Answer from the drawing. Dimensions are ordinates in mm from the lowest x, y and z of the part. Give positions to 0.01 mm unless a question says otherwise; leave off trailing zeros. Write each loop counter-clockwise with the first axis right and the second up, starting at its lowest first coordinate (ties: lowest second). Pieces come first, ordered by that corner, then holes.
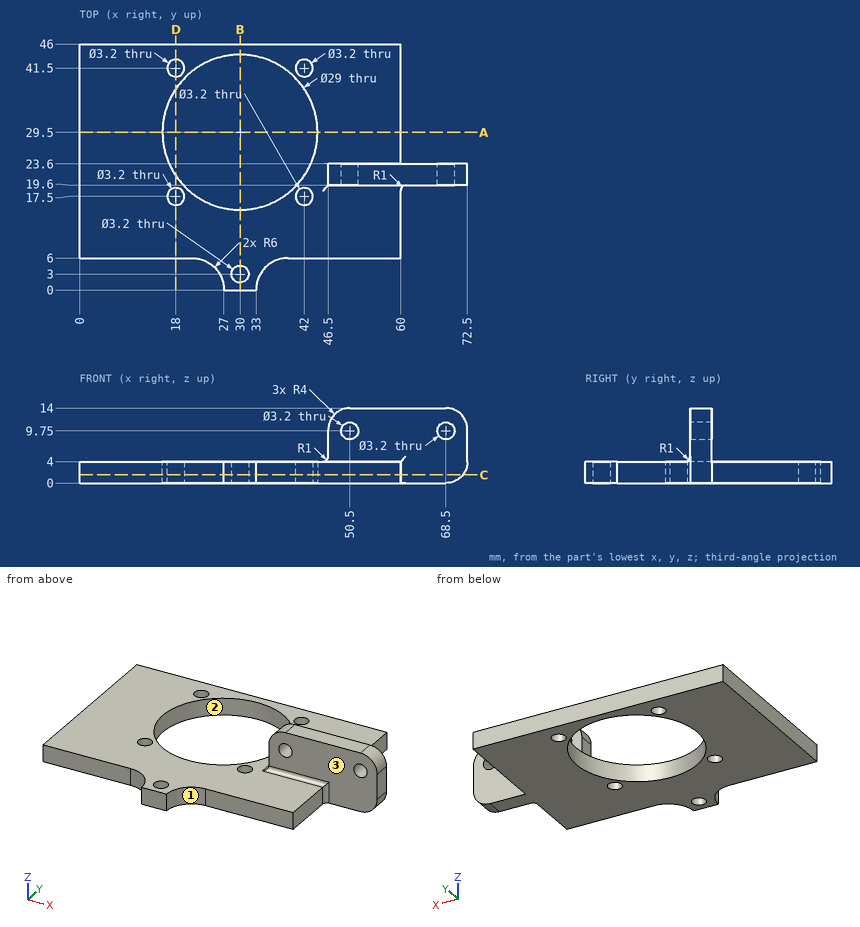
Item 1: A cutting plane is placed at C-C, the plane z = 1.5. Count the separate pieces of the cut face and the enclosed holes in it, plus the area to 3 significant figures.
Conclusion:
separate pieces: 1
enclosed holes: 6
area: 1,800 mm2
Item 2: Each of these flat-tipped pins is pushed along its axis until it touches: P1, Ø5, axis at x = 42, y = 41.5, coming from the +Z side; P2, Ø1.5, axis at y = 24, z = 3, coming from the +X side; P3, Ø2, axis at y = 34, z = 1, coming from the +X side. Where does it stop, or does it pass through?
Conclusion:
P1: stops at z = 4
P2: stops at x = 72.48
P3: stops at x = 60
Item 3: Consider probe 1 along Y at (x, z) = (30, 2.25); probe 2 along X at (y, z) = (22.15, 9.75); probe 3 along Y at (x, z) = (42, 1.9). Determine where each line is inside the solid, lowest interval first.
Conclusion:
probe 1: y = 0 to 1.4, 4.6 to 15, 44 to 46
probe 2: x = 46.5 to 48.9, 52.1 to 66.9, 70.1 to 72.5
probe 3: y = 6 to 15.9, 19.1 to 21.36, 37.64 to 39.9, 43.1 to 46
Item 4: A cutting plane is placed at A-A, the plane y = 29.5. Give the vertices of the cut face in (x, z), plus the area to 3 significant figures.
Conclusion:
outline: (0, 0) - (15.5, 0) - (15.5, 4) - (0, 4) - close; (44.5, 0) - (60, 0) - (60, 4) - (44.5, 4) - close
area: 124 mm2
Item 5: A cutting plane is placed at B-B, the plane x = 30. Give the vertices of the cut face in (y, z).
Conclusion:
outline: (0, 0) - (1.4, 0) - (1.4, 4) - (0, 4) - close; (4.6, 0) - (15, 0) - (15, 4) - (4.6, 4) - close; (44, 0) - (46, 0) - (46, 4) - (44, 4) - close
Item 6: A cutting plane is placed at D-D, the plane x = 18. Give the vertices of the cut face in (y, z), plus the area to 3 significant figures.
Conclusion:
outline: (6, 0) - (15.9, 0) - (15.9, 4) - (6, 4) - close; (19.1, 0) - (21.36, 0) - (21.36, 4) - (19.1, 4) - close; (37.64, 0) - (39.9, 0) - (39.9, 4) - (37.64, 4) - close; (43.1, 0) - (46, 0) - (46, 4) - (43.1, 4) - close
area: 69.3 mm2
Item 7: Determine the mould class of the marked faces 1, 2 and 3 for opening direction X: pulls with the +X half, pulls with the -X half, needs draft (parallel to the pull), parting line crosses it, or undercut.
Conclusion:
face 1: pulls with the +X half
face 2: undercut
face 3: needs draft
